The model under review builds one solid part; all positions refer to its coordinate system, in mm. A direction names the side the tool comes from. Coordinates: 2 decimals unless noted, no trailing zeros. Write each loop counter-clockwise with the first axis right and the second up, starting at its lowest first coordinate (ties: lowest second). Pieces come first, ordered by that corner, then holes. Notation, with made-up numbers: (65.5, 46) - (109.5, 46) arc R19 ccw to (109.5, 52) - close; hole circle Ø7 at (64, 37.25). An arc over 180 degrees is marked (long way). Return JSON: item names as keys, results as strings. Group by question number.
(1) To check wall thickness, follow L1, parallel to Y at x = 0, z = 7.7 (1 decimal); L2, parallel to Z at x = 11, y = 2.5 (3 decimals); L3, parallel to Y at x = 0, z = 0.55 (1 decimal). State the ranges of each line that lie inside material, in increasing order. Write a range as from..to.
(2) For pin 1 Ø3 at (y, z) = (1.5, 1) entering from +X; pin 2 Ø3 at (y, z) = (10.5, 4) entering from -X, all flat-tipped, find the tip position at first contact; note any pin that passes through.
(3) We need section A-A on z = 5.5. State the section outline as (x, y) points (1 decimal).
(4) Draft analysis for pull direction X (two halves, no side actions). For faces 1 (the face through (0.39, 6.34, 3.91)), 2 (the face through (2.3, 6.5, 0)), 3 (the face through (-14.274, -0.628, 3.239)), state which applies: released by +X, released by -X, zero draft, split by the parting line, or undercut.
(5) Tool access review of faces 4 (the face through (5.491, -10.557, 7.614)), 5 (the face through (2, -14, 6.403)), 6 (the face through (-5.7, -2.8, 3.9)), 7 (the face through (7.559, -5.796, 0.313)): name each direction out of +Z, -Z, +X, -X, +Y, -Y from which nothing blocks a thin tool from reaching the whole face with its end or side.
```python
from build123d import *

# Parameters (mm, degrees)
CHAMFER1_SIZE       = 0.127
FILLET2_R           = 0.508
CUT_EXTRUDE2_REACH  = 9.927
SKETCH3_R           = 11.899111158
SKETCH4_R           = 9.525
BOSS_EXTRUDE1_DEPTH = 7.92734
SKETCH5_R           = 11.899111158
SKETCH5_R_2         = 9.525
BOSS_EXTRUDE2_DEPTH = 6.65734


with BuildPart() as part:
    # Sketch1 → Revolve1 (revolve)
    with BuildSketch(Plane.XZ):
        Polygon((15.4305, 7.92734), (0, 7.92734), (0, 0), (14.2875, 0), (14.2875, 5.89534), (13.97, 5.89534), (13.97, 6.40334), (15.5575, 6.40334), (15.5575, 7.80034), align=None)
    revolve(axis=Axis((0, 0, 7.92734), (0, 0, -1)))

    # Chamfer1
    chamfer1_edges = [part.edges().sort_by_distance(p)[0] for p in [
        (-15.5575, 0, 6.40334),
    ]]
    chamfer(chamfer1_edges, length=CHAMFER1_SIZE)

    # Fillet2
    fillet2_edges = [part.edges().sort_by_distance(p)[0] for p in [
        (-14.2875, 0, 0),
    ]]
    fillet(fillet2_edges, radius=FILLET2_R)

    # Sketch3 → Cut-Extrude2 (cut, up to next)
    with BuildSketch(Plane.XY.offset(7.92734), mode=Mode.PRIVATE) as cut_extrude2_sk1:
        Circle(SKETCH3_R)
    cut_extrude2_tool1 = extrude(cut_extrude2_sk1.sketch, amount=-CUT_EXTRUDE2_REACH, mode=Mode.PRIVATE) & part.part
    add(cut_extrude2_tool1.solids().sort_by_distance((0, 0, 7.92734))[0], mode=Mode.SUBTRACT)



with BuildPart() as body_2:
    # Sketch4 → Boss-Extrude1 (new body)
    with BuildSketch(Plane(origin=(0, 0, 0), x_dir=(-1, 0, 0), z_dir=(0, 0, -1))):
        Circle(SKETCH4_R)
        Polygon((-3.212275886, -6.591253065), (4.102054654, -6.077539054), (7.31433054, 0.513714011), (3.212275886, 6.591253065), (-4.102054654, 6.077539054), (-7.31433054, -0.513714011), align=None, mode=Mode.SUBTRACT)
    extrude(amount=-BOSS_EXTRUDE1_DEPTH)


with BuildPart() as part_1:
    add(part.part)

    add(body_2.part)  # Boss-Extrude2 merges body 2
    # Sketch5 → Boss-Extrude2 (add)
    with BuildSketch(Plane(origin=(0, 0, 0.635), x_dir=(-1, 0, 0), z_dir=(0, 0, -1))):
        Circle(SKETCH5_R)
        Circle(SKETCH5_R_2, mode=Mode.SUBTRACT)
    extrude(amount=-BOSS_EXTRUDE2_DEPTH)


solid = part_1.part
```
Ans:
{
 "1": {"L1": "-15.6..-11.9, -9.5..-6.4, 6.4..9.5, 11.9..15.6", "L2": "0.635..7.292", "L3": "-14.3..-11.9, -9.5..-6.4, 6.4..9.5, 11.9..14.3"},
 "2": {"pin 1": "x = 14.29", "pin 2": "x = -11.1"},
 "3": {"outline": "circle Ø28.6 at (0, 0); hole (-7.3, 0.5) - (-4.1, -6.1) - (3.2, -6.6) - (7.3, -0.5) - (4.1, 6.1) - (-3.2, 6.6) - close"},
 "4": {"face 1": "undercut", "face 2": "zero draft", "face 3": "split by the parting line"},
 "5": {"face 4": "+Z", "face 5": "none", "face 6": "+Z, -Z", "face 7": "-Z"}
}
